The figure shows three views and two pictorial views of one solid part (mm, origin at its lowest corner). Answer the questions. Coordinates: 2 decimals unless noted, no trailing zeros. Write each loop counter-clockwise with the first axis right and the second up, starting at its lowest first coordinate (ties: lowest second). Pieces come first, ordered by that corner, then holes. Notation, with made-up numbers: (23.5, 47) - (29.5, 47) arc R13 ccw to (29.5, 63) - close; hole circle Ø11 at (47, -38.5). An arc over 180 degrees is marked (long way). Use a Markdown table: item, result. Add a question column.
(1) The part is cut by section B-B, the plane y = 1.25. Give the vertices of the cut face in (x, z).
(2) The part is cut by section D-D, the plane y = 8.5. Give the vertices of the cut face in (x, z) (1 decimal).
(3) Given pin 1 Ø1.9 at (x, y) = (4.76, 4.76) entering from -Z; pin 2 Ø4 at (y, z) = (2, 43.5) entering from -X; pin 3 Ø2 at (x, z) = (7, 45) entering from +Y, each flat-ended and moving along its own axis, determine where each tip first touches the part or whether it passes through.
(4) Find the intervals of material crossed by line 1 (X direction, y = 4, z = 56.5) (1 decimal); line 2 (Y direction, x = 5, z = 17.5) (1 decimal); line 3 (Y direction, x = 3.25, z = 40.5) (1 decimal), in increasing order. Write a range as from..to.
(5) The part is cut by section A-A, the plane x = 5.5. Give the vertices of the cut face in (y, z).
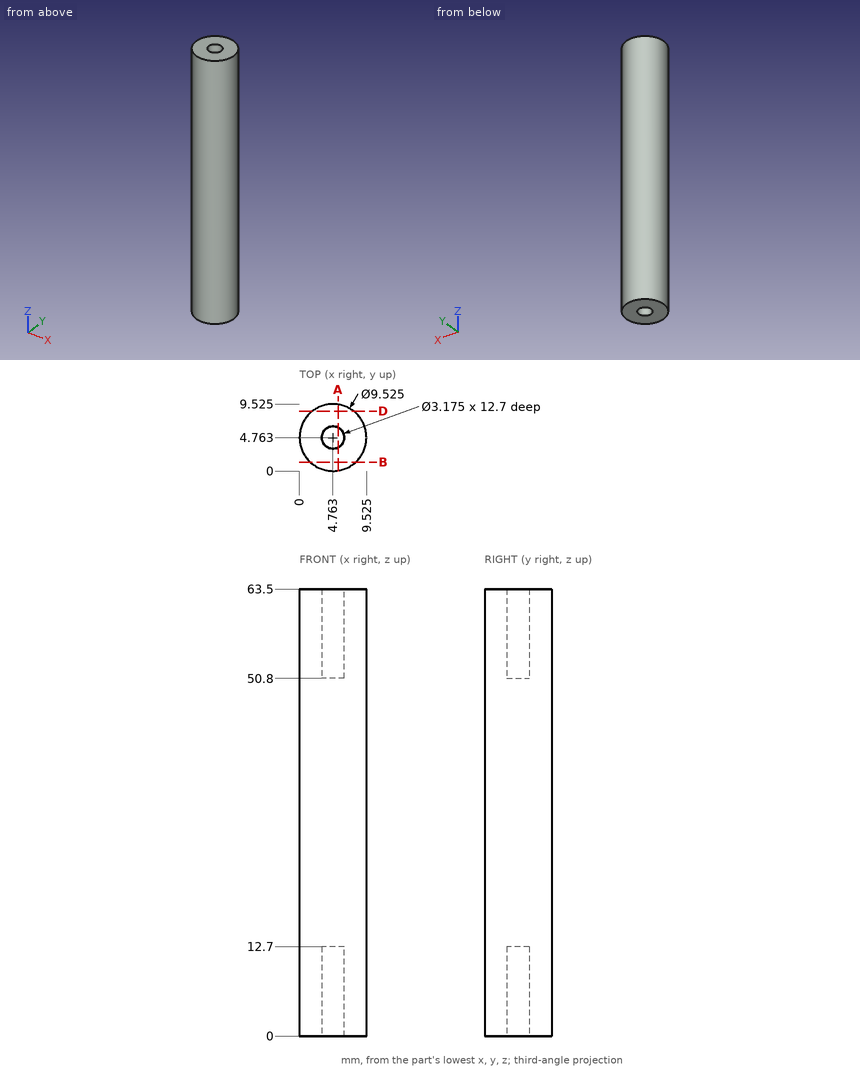
Model answer:
| question | item | result |
|---|---|---|
| 1 | outline | (1.55, 0) - (7.98, 0) - (7.98, 63.5) - (1.55, 63.5) - close |
| 2 | outline | (1.8, 0) - (7.7, 0) - (7.7, 63.5) - (1.8, 63.5) - close |
| 3 | pin 1 | z = 12.7 |
| 3 | pin 2 | x = 0.06 |
| 3 | pin 3 | y = 9.36 |
| 4 | line 1 | 0.1..3.4, 6.2..9.5 |
| 4 | line 2 | 0..9.5 |
| 4 | line 3 | 0.2..9.3 |
| 5 | outline | (0.06, 0) - (3.36, 0) - (3.36, 12.7) - (6.17, 12.7) - (6.17, 0) - (9.47, 0) - (9.47, 63.5) - (6.17, 63.5) - (6.17, 50.8) - (3.36, 50.8) - (3.36, 63.5) - (0.06, 63.5) - close |
